Read the model definition and answer for the solid it produces. Units are mm, in the model's axes. A direction names the side the tool comes from. Give positions to 0.01 mm unless a question says otherwise; leave off trailing zeros. Order: outer loops, then holes, each group sorted by start corner. A loop starts at its lowest first (then second) coordinate and runs counter-clockwise, first axis right, second up.
```python
from build123d import *

# Parameters (mm, degrees)
BOSS_EXTRUDE2_DEPTH = 50.8
SKETCH3_R           = 1.75
CUT_EXTRUDE1_DEPTH  = 76.2
SKETCH4_R           = 2.15
SKETCH4_W           = 6.35
SKETCH4_H           = 12.7
CUT_EXTRUDE2_DEPTH  = 76.2
SKETCH6_R           = 1.75
CUT_EXTRUDE3_DEPTH  = 76.2
SKETCH7_R           = 2.15
SKETCH7_W           = 6
SKETCH7_H           = 12.7
CUT_EXTRUDE4_DEPTH  = 76.2
FILLET1_R           = 1


with BuildPart() as part:
    # Sketch2 → Boss-Extrude2 (new body)
    with BuildSketch(Plane(origin=(0, 0, 0), x_dir=(0, 1, 0), z_dir=(0, 0, 1))):
        Polygon((0, 0), (-17.78, 0), (-17.78, 7.62), (-7.62, 7.62), (-7.62, 17.78), (0, 17.78), align=None)
    extrude(amount=BOSS_EXTRUDE2_DEPTH)

    # Sketch3 → Cut-Extrude1 (cut)
    with BuildSketch(Plane(origin=(0, 0, 0), x_dir=(-1, 0, 0), z_dir=(0, 1, 0))):
        with Locations((4.36625, 15.875)):
            Circle(SKETCH3_R)
    extrude(amount=-CUT_EXTRUDE1_DEPTH, mode=Mode.SUBTRACT)

    # Sketch4 → Cut-Extrude2 (cut)
    with BuildSketch(Plane(origin=(-7.62, 0, 0), x_dir=(0, -1, 0), z_dir=(-1, 0, 0))):
        with Locations(Location((12.54125, 5.08, 0), (0, 0, 90))):
            Circle(SKETCH4_R)
        with Locations(Location((12.54125, 45.72, 0), (0, 0, 90))):
            Circle(SKETCH4_R)
        with Locations((11.366242, 15.875)):
            Rectangle(SKETCH4_W, SKETCH4_H)
    extrude(amount=-CUT_EXTRUDE2_DEPTH, mode=Mode.SUBTRACT)

    # Sketch6 → Cut-Extrude3 (cut)
    with BuildSketch(Plane(origin=(-17.78, 0, 0), x_dir=(0, -1, 0), z_dir=(-1, 0, 0))):
        with Locations(Location((4.36626, 28.575, 0), (0, 0, 90))):
            Circle(SKETCH6_R)
    extrude(amount=-CUT_EXTRUDE3_DEPTH, mode=Mode.SUBTRACT)

    # Sketch7 → Cut-Extrude4 (cut)
    with BuildSketch(Plane.XZ.offset(7.62)):
        with Locations((-12.54125, 45.72)):
            Circle(SKETCH7_R)
        with Locations((-12.54125, 5.08)):
            Circle(SKETCH7_R)
        with Locations((-11.541246, 28.575)):
            Rectangle(SKETCH7_W, SKETCH7_H)
    extrude(amount=-CUT_EXTRUDE4_DEPTH, mode=Mode.SUBTRACT)

    # Fillet1
    fillet1_edges = [part.edges().sort_by_distance(p)[0] for p in [
        (-3.81, -8.191242, 22.225),
        (-3.81, -14.541242, 9.525),
        (-3.81, -8.191242, 9.525),
        (-3.81, -14.541242, 22.225),
        (-14.541246, -3.81, 34.925),
        (-8.541246, -3.81, 22.225),
        (-14.541246, -3.81, 22.225),
        (-8.541246, -3.81, 34.925),
    ]]
    fillet(fillet1_edges, radius=FILLET1_R)


solid = part.part
```
1) The part is cut by section A-A on z = 45.72. Determine the outline of the cut face in (x, y).
Final values:
outline: (-17.78, -7.62) - (-14.69, -7.62) - (-14.69, 0) - (-17.78, 0) - close; (-10.39, -7.62) - (-7.62, -7.62) - (-7.62, -10.39) - (0, -10.39) - (0, 0) - (-10.39, 0) - close; (-7.62, -17.78) - (0, -17.78) - (0, -14.69) - (-7.62, -14.69) - close
2) A tool of negligible diameter and unlimited length cuts with its end or side. For faces 1 (the face through (-4, -17.78, 25)), 2 (the face through (-14.24, -3.76, 34.64)), 3 (the face through (-4, -11, 22.225)), 4 (the face through (-15, -7.62, 25)), from which of +Z, -Z, +X, -X, +Y, -Y can it reach the whole face along a straight path? Write none if from no direction.
Final values:
face 1: +Z, -Z, +X, -X, -Y
face 2: +Y, -Y
face 3: +X, -X
face 4: +Z, -Z, -X, -Y
3) For a pull along Z with two mould halves and no side action, classify faces 5 (the face through (-7, -7, 50.8)), 6 (the face through (-11.385, -3.863, 47.533)), 7 (the face through (-7.62, -13, 25)) as released by +Z, released by -Z, zero draft, split by the parting line, or undercut.
Final values:
face 5: released by +Z
face 6: undercut
face 7: zero draft
4) The part is cut by section D-D on x = -4.75. Determine the outline of the cut face in (y, z) (3 decimals), and give its area (3 significant figures).
Final values:
outline: (-17.78, 0) - (0, 0) - (0, 14.168) - (-8.191, 14.168) - (-8.191, 10.525) arc R1 cw to (-9.191, 9.525) - (-13.541, 9.525) arc R1 cw to (-14.541, 10.525) - (-14.541, 14.168) - (-17.78, 14.168) - close; (-17.78, 17.582) - (-14.541, 17.582) - (-14.541, 21.225) arc R1 cw to (-13.541, 22.225) - (-9.191, 22.225) arc R1 cw to (-8.191, 21.225) - (-8.191, 17.582) - (0, 17.582) - (0, 50.8) - (-17.78, 50.8) - close; hole circle Ø4.3 at (-12.541, 5.08); hole circle Ø4.3 at (-12.541, 45.72); hole circle Ø3.5 at (-4.366, 28.575)
area: 746 mm2
5) Given pin 1 (1.5 mm diameter, centred on x = -7.5, z = 32.5, fed in from +Y); pin 2 (2 mm diameter, centred on y = -4.37, z = 28.58, fed in from -X); pin 3 (7 mm diameter, centred on x = -12.54, z = 5.08, fed in from -Y), each flat-ended and moving along its own axis, determine where each tip first touches the part or whether it passes through.
Final values:
pin 1: stops at y = 0
pin 2: passes through
pin 3: stops at y = -7.62
6) Consider L1, parallel to Y at x = -6, z = 5.08; L2, parallel to Y at x = -6.75, z = 13.5; L3, parallel to Z at x = -6.5, y = -10 (3 decimals). Determine where each line is inside the solid, lowest interval first.
Final values:
L1: y = -17.78 to -14.69, -10.39 to 0
L2: y = -17.78 to -14.54, -8.19 to 0
L3: z = 0 to 9.525, 22.225 to 50.8
7) The part is cut by section B-B on y = -3.5. Determine the outline of the cut face in (x, z) (3 decimals), and give its area (3 significant figures).
Final values:
outline: (-17.78, 0) - (0, 0) - (0, 27.054) - (-8.541, 27.054) - (-8.541, 23.225) arc R1 cw to (-9.541, 22.225) - (-13.541, 22.225) arc R1 cw to (-14.541, 23.225) - (-14.541, 27.054) - (-17.78, 27.054) - close; (-17.78, 30.096) - (-14.541, 30.096) - (-14.541, 33.925) arc R1 cw to (-13.541, 34.925) - (-9.541, 34.925) arc R1 cw to (-8.541, 33.925) - (-8.541, 30.096) - (0, 30.096) - (0, 50.8) - (-17.78, 50.8) - close; hole circle Ø4.3 at (-12.541, 5.08); hole circle Ø4.3 at (-12.541, 45.72); hole circle Ø3.5 at (-4.366, 15.875)
area: 753 mm2
8) The part is cut by section C-C on z = 11.5. Determine the outline of the cut face in (x, y).
Final values:
outline: (-17.78, -7.62) - (-7.62, -7.62) - (-7.62, -8.19) - (0, -8.19) - (0, 0) - (-17.78, 0) - close; (-7.62, -17.78) - (0, -17.78) - (0, -14.54) - (-7.62, -14.54) - close
